Drawing for the job (mm, zero at the part's lowest x, y, z). A direction names the side the tool comes from. Round coordinates to 2 decimals unless told otherwise and drop trailing zeros. Write each loop counter-clockwise with the first axis right and the second up, starting at its lowest first coordinate (ties: lowest second). Pieces come first, ordered by that corner, then holes.
Item 1: Band-saw the part on C-C, the plane x = 9. Write the cut outline in (y, z), then the cut area to 3 significant figures.
Item 2: Band-saw the part on A-A, the plane y = 27. Write the cut outline in (x, z).
Item 3: Band-saw the part on D-D, the plane y = 37.5. Write the cut outline in (x, z).
Item 4: 3-axis set-ups, long thin cutter, end or side, ignore diameter. For the marked faces 5 and 6: which of +Z, -Z, +X, -X, +Y, -Y reach the whole face in a straight line?
Item 5: Drop flat-ended pins along their axis: pin 1 Ø4 at (x, z) = (9, 95) entering from +Y; pin 2 Ø1 at (x, z) = (43, 65.5) entering from +Y; pin 3 Ø11 at (x, z) = (114, 75.5) entering from +Y. Give the stop position or say it passes through.
Item 6: Wall check: probe 1 along Z at (x, y) = (109, 40.25); probe 2 along X at (y, z) = (39.25, 9); probe 3 along Z at (x, y) = (54.5, 7.5). Give the ranges that are in metal, low to high.
Item 7: Mould opens along X. For the marked faces 1, 2, 3 and 4 say: +X half, -X half, draft (parallel to the pull), parting line (faces both ways), or undercut.
Item 8: Band-saw the part on B-B, the plane z = 9. Write the cut outline in (x, y), then the cut area to 3 significant figures.
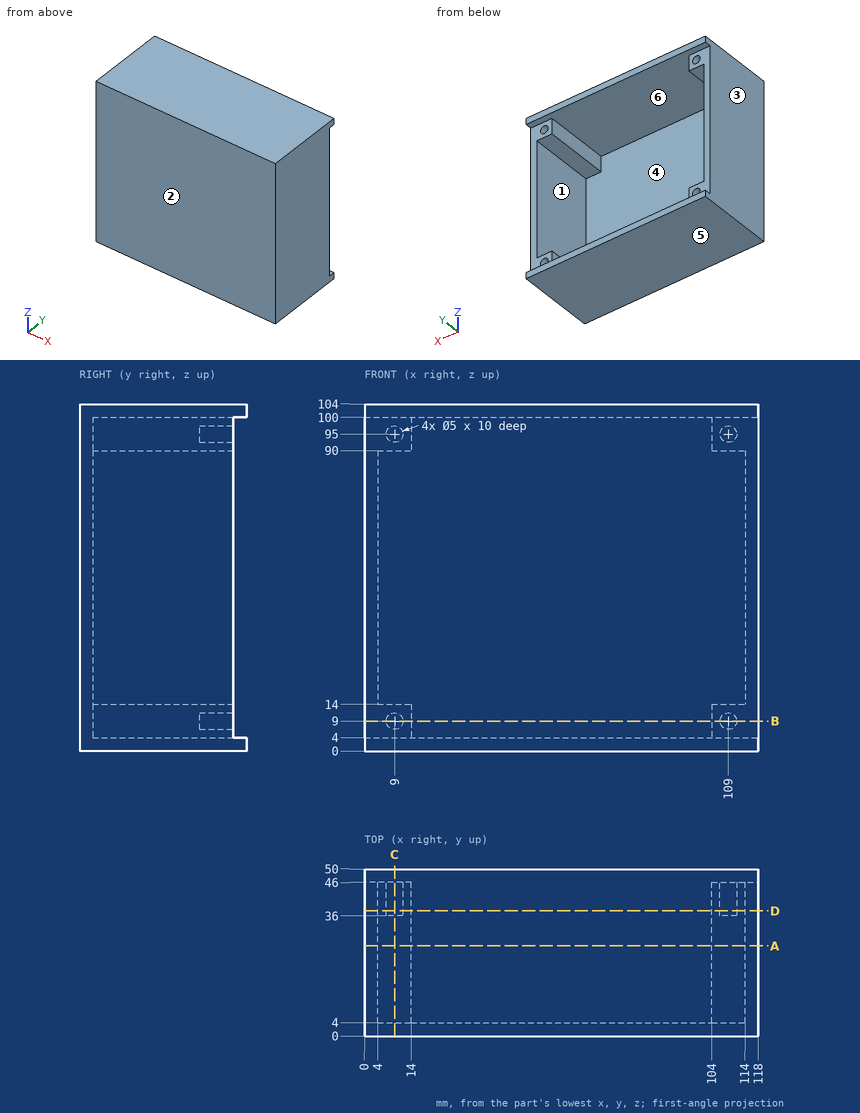
Results:
1. outline: (0, 0) - (50, 0) - (50, 4) - (46, 4) - (46, 6.5) - (36, 6.5) - (36, 11.5) - (46, 11.5) - (46, 14) - (4, 14) - (4, 90) - (46, 90) - (46, 92.5) - (36, 92.5) - (36, 97.5) - (46, 97.5) - (46, 100) - (50, 100) - (50, 104) - (0, 104) - close
1. area: 1,520 mm2
2. outline: (0, 0) - (118, 0) - (118, 104) - (0, 104) - close; hole (4, 14) - (14, 14) - (14, 4) - (104, 4) - (104, 14) - (114, 14) - (114, 90) - (104, 90) - (104, 100) - (14, 100) - (14, 90) - (4, 90) - close
3. outline: (0, 0) - (118, 0) - (118, 104) - (0, 104) - close; hole (4, 14) - (14, 14) - (14, 4) - (104, 4) - (104, 14) - (114, 14) - (114, 90) - (104, 90) - (104, 100) - (14, 100) - (14, 90) - (4, 90) - close; hole circle Ø5 at (9, 9); hole circle Ø5 at (9, 95); hole circle Ø5 at (109, 9); hole circle Ø5 at (109, 95)
4. face 5: -Z, +X, -X, +Y, -Y
4. face 6: +Y
5. pin 1: stops at y = 36
5. pin 2: stops at y = 4
5. pin 3: stops at y = 46
6. probe 1: z = 0 to 6.5, 11.5 to 14, 90 to 92.5, 97.5 to 104
6. probe 2: x = 0 to 6.5, 11.5 to 14, 104 to 106.5, 111.5 to 118
6. probe 3: z = 0 to 4, 100 to 104
7. face 1: undercut
7. face 2: draft
7. face 3: -X half
7. face 4: undercut
8. outline: (0, 0) - (118, 0) - (118, 46) - (111.5, 46) - (111.5, 36) - (106.5, 36) - (106.5, 46) - (104, 46) - (104, 4) - (14, 4) - (14, 46) - (11.5, 46) - (11.5, 36) - (6.5, 36) - (6.5, 46) - (0, 46) - close
8. area: 1,550 mm2
